Could you check a few things on this drawing? It's one solid part, dimensions in mm from its lowest x, y, z. A direction names the side the tool comes from. Give positions to 0.01 mm unless a question says otherwise; leave off trailing zeros. Order: outer loops, then holes, each group sorted by start corner. A loop starts at its lowest first (then second) coordinate and runs counter-clockwise, first axis right, second up. Notation, with made-up numbers: M -25.75,37.5 L -10.75,37.5 A16 ccw -10.75,54.5 Z; hole C -26.75,-23.75 d11. An arc over 180 degrees is marked long. Use one line per item in the form item = value.
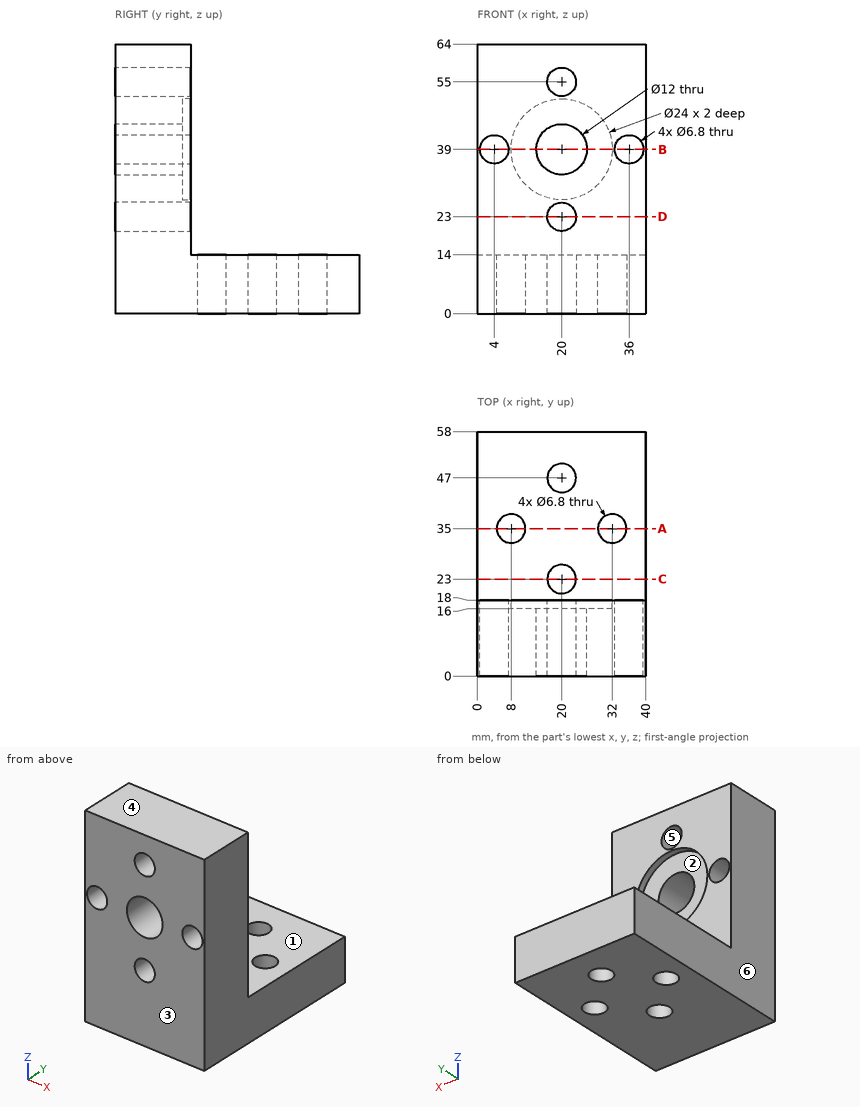
Q1. I want a section at D-D on z = 23. Write out the boundary of the cut face in (x, y), then the cut area to 3 significant figures.
Found:
outline = M 0,0 L 16.6,0 L 16.6,18 L 0,18 Z; M 23.4,0 L 40,0 L 40,18 L 23.4,18 Z
area = 598 mm²
Q2. I want a section at B-B on z = 39. Write out the boundary of the cut face in (x, y).
Found:
outline = M 0,0 L 0.6,0 L 0.6,18 L 0,18 Z; M 7.4,0 L 14,0 L 14,16 L 8,16 L 8,18 L 7.4,18 Z; M 26,0 L 32.6,0 L 32.6,18 L 32,18 L 32,16 L 26,16 Z; M 39.4,0 L 40,0 L 40,18 L 39.4,18 Z
Q3. On a 3-axis mill with a long thin cutter (end or side, diameter ignored), from which of +Z, -Z, +X, -X, +Y, -Y can I reach the whole of each face in a straight line? I mean the marked faces 1, 2 and 3. Say none if no direction works.
Found:
face_1 = +Z, +X, -X, +Y
face_2 = +Y
face_3 = +Z, -Z, +X, -X, -Y
Q4. I want a section at A-A on y = 35. Write out the boundary of the cut face in (x, z), then the cut area to 3 significant figures.
Found:
outline = M 0,0 L 4.6,0 L 4.6,14 L 0,14 Z; M 11.4,0 L 28.6,0 L 28.6,14 L 11.4,14 Z; M 35.4,0 L 40,0 L 40,14 L 35.4,14 Z
area = 370 mm²
Q5. I'm going to push flat-ended pins straight in: pin 1 Ø11 at (x, z) = (20, 55) entering from -Y; pin 2 Ø7 at (x, z) = (22.5, 44) entering from +Y; pin 3 Ø4 at (x, z) = (8.5, 24.5) entering from +Y. Where does each tip first touch, or does it pass through?
Found:
pin_1 = 0
pin_2 = 16
pin_3 = 18
Q6. Thinking about a two-plate mould opening in X: for the marked faces 4, 5 and 6, which applies, +X half, -X half, draft (parallel to the pull), parting line (faces both ways), or undercut?
Found:
face_4 = draft
face_5 = undercut
face_6 = -X half
Q7. I need wall thicknesses on L1, parallel to Y at x = 20, z = 9; L2, parallel to X at y = 13, z = 39; L3, parallel to X at y = 17.55, z = 39. Which ranges of each line are inside material? Lowest first, please.
Found:
L1 = 0 to 19.6, 26.4 to 43.6, 50.4 to 58
L2 = 0 to 0.6, 7.4 to 14, 26 to 32.6, 39.4 to 40
L3 = 0 to 0.6, 7.4 to 8, 32 to 32.6, 39.4 to 40
Q8. I want a section at C-C on y = 23. Write out the boundary of the cut face in (x, z), then the cut area to 3 significant figures.
Found:
outline = M 0,0 L 16.6,0 L 16.6,14 L 0,14 Z; M 23.4,0 L 40,0 L 40,14 L 23.4,14 Z
area = 465 mm²
